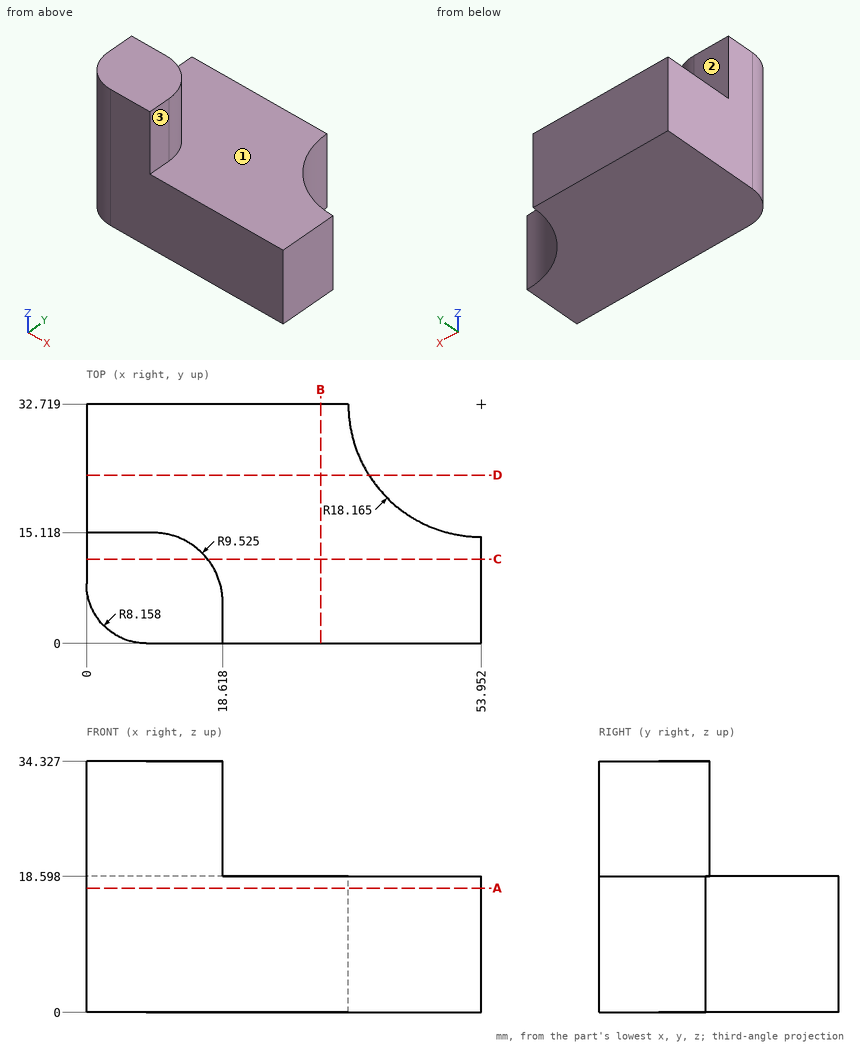
Could you check a few things on this drawing? It's one solid part, dimensions in mm from its lowest x, y, z. A direction names the side the tool comes from. Coordinates: 2 decimals unless noted, no trailing zeros. Order: outer loops, then holes, each group sorted by start corner. A loop starts at its lowest first (then second) coordinate and runs counter-clockwise, first axis right, second up. Notation, with made-up numbers: (68, 78) - (110, 78) arc R22 cw to (110, 97) - close; hole circle Ø11 at (-30, 67). An arc over 180 degrees is marked (long way). Answer as a JSON object with one key per item and string values. Group by question number.
Q1. Will these pins go through, and if not, where does the flat tip stop? P1, Ø4, axis at y = 5, z = 30, coming from the +X side; P2, Ø6, axis at x = 13.5, y = 25.5, coming from the +Z side; P3, Ø4.5, axis at x = 4, z = 25.5, coming from the +Y side.
Q2. Imagine slicing it at B-B (x = 32). Please give me the cut outline in (y, z).
Q3. Imagine slicing it at C-C (y = 11.5). Please give me the cut outline in (x, z) (1 decimal).
Q4. Imagine slicing it at A-A (z = 17). Please give me the cut outline in (x, y) (1 decimal).
Q5. On a 3-axis mill with a long thin cutter (end or side, diameter ignored), from which of +Z, -Z, +X, -X, +Y, -Y can I reach the whole of each face in a straight line? I mean the marked faces 1, 2 and 3. Say none if no direction works.
Q6. I need wall thicknesses on line 1 (Z direction, x = 12, y = 19.5); line 2 (Y direction, x = 52, z = 13); line 3 (X direction, y = 23, z = 5) (1 decimal). Which ranges of each line are inside material? Lowest first, please. Write a range as from..to.
Q7. Imagine slicing it at D-D (y = 23). Please give me the cut outline in (x, z), and give its area (3 significant figures).
Determined:
{
 "1": {"P1": "stops at x = 18.62", "P2": "stops at z = 18.6", "P3": "stops at y = 15.12"},
 "2": {"outline": "(0, 0) - (32.72, 0) - (32.72, 18.6) - (0, 18.6) - close"},
 "3": {"outline": "(0, 0) - (54, 0) - (54, 18.6) - (16.6, 18.6) - (16.6, 34.3) - (0, 34.3) - close"},
 "4": {"outline": "(0, 8.2) arc R8.2 ccw to (8.2, 0) - (54, 0) - (54, 14.6) arc R18.2 cw to (35.8, 32.7) - (0, 32.7) - close"},
 "5": {"face 1": "+Z, +X, +Y", "face 2": "+Z, +X, -X, +Y", "face 3": "+Z, +X, +Y, -Y"},
 "6": {"line 1": "z = 0..18.6", "line 2": "y = 0..14.66", "line 3": "x = 0..38.6"},
 "7": {"outline": "(0, 0) - (38.61, 0) - (38.61, 18.6) - (0, 18.6) - close", "area": "718 mm2"}
}
